The figure shows three views and two pictorial views of one solid part (mm, origin at its lowest corner). Answer the questions. Coordinates: 2 decimals unless noted, no trailing zeros. Write each loop counter-clockwise with the first axis right and the second up, starting at its lowest first coordinate (ties: lowest second). Pieces come first, ordered by that corner, then holes.
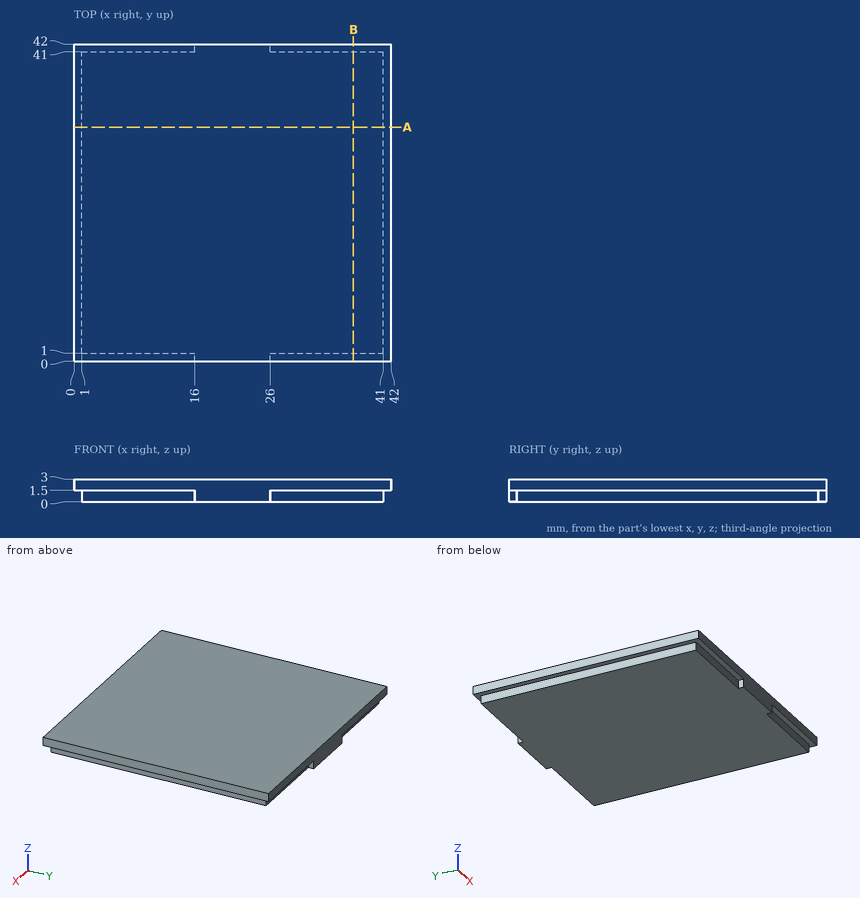
Item 1: The part is cut by section A-A (y = 31). Give the vertices of the cut face in (x, z), and give its area (3 significant figures).
Item 2: Find the intervals of material crossed by probe 1 along X at (y, z) = (9, 0.8), in increasing order.
Item 3: Given pin 1 (0.8 mm diameter, centred on x = 6.5, z = 0.5, fed in from +Y); pin 2 (1.6 mm diameter, centred on x = 36.5, z = 0.5, fed in from -Y); pin 3 (0.5 mm diameter, centred on y = 0.5, z = 1, fed in from -X), each flat-ended and moving along its own axis, determine where each tip first touches the part or whether it passes through.
Answer:
1. outline: (0, 1.5) - (1, 1.5) - (1, 0) - (41, 0) - (41, 1.5) - (42, 1.5) - (42, 3) - (0, 3) - close
1. area: 123 mm2
2. probe 1: x = 1 to 41
3. pin 1: stops at y = 41
3. pin 2: stops at y = 1
3. pin 3: stops at x = 16
